Read the model definition and answer for the solid it produces. Units are mm, in the model's axes. Face numbers are marked on the shaded views. A direction names the side the tool comes from. Round coordinates to 2 decimals unless told otherwise and drop trailing zeros. Order: outer loops, then holes, each group sorted by start corner. A loop starts at its lowest first (then second) coordinate and runs counter-clockwise, first axis right, second up. Notation, with made-up numbers: (81, -26) -> (101, -26) arc R11 cw to (101, -13) -> close; hole circle Ø5 at (22.5, -23.5). An arc over 180 degrees is marked (long way). Use a Markdown table: item, result. Add a question column.
1. Consider L1, parallel to Y at x = 0, z = 8.75; L2, parallel to Z at x = -9.5, y = 2; L3, parallel to Z at x = 0.75, y = 2.25. Determine where each line is inside the solid, lowest interval first. Write a range as [from, to].
2. Section B-B, the plane z = -22.5 is taken. Give the vertices of the cut face in (x, y), then the cut area to 3 significant figures.
3. The mould has two halves that part along X. Classify the marked faces 3, 4 and 5: +X half, -X half, draft (parallel to the pull), parting line (faces both ways), or undercut.
4. For the marked faces 1 and 2, determine the directions among +Z, -Z, +X, -X, +Y, -Y from which every point of the face is accessible in a straight line to the end or side of a thin tool.
5. Given pin 1 (6 mm diameter, centred on y = 2.5, z = -12.5, fed in from +X); pin 2 (6 mm diameter, centred on x = -6, z = -24, fed in from +Y); pin 3 (1 mm diameter, centred on x = -3, z = 9.5, fed in from +Y), each flat-ended and moving along its own axis, determine where each tip first touches the part or whether it passes through.
6. Section A-A, the plane z = 15 is taken. Give the vertices of the cut face in (x, y).
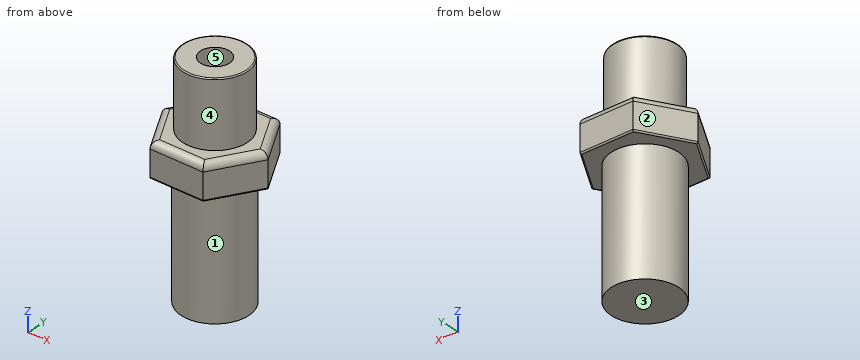
Autodesk Inventor part; units mm, degrees
ref_plane "YZ Plane" through (0, 0, 0) normal (1, 0, 0) x (0, 1, 0)
ref_plane "XZ Plane" through (0, 0, 0) normal (0, 1, 0) x (-1, 0, 0)
ref_plane "XY Plane" through (0, 0, 0) normal (0, 0, 1) x (1, 0, 0)
sketch "Sketch1" plane through (0, 0, 0) normal (0, 0, 1) x (1, 0, 0)
  line L0 (6.4577, 10.7072) -> (12.5016, -0.2389)
  line L1 (12.5016, -0.2389) -> (6.0439, -10.9461)
  line L2 (6.0439, -10.9461) -> (-6.4577, -10.7072)
  line L3 (-6.4577, -10.7072) -> (-12.5016, 0.2389)
  line L4 (-12.5016, 0.2389) -> (-6.0439, 10.9461)
  line L5 (-6.0439, 10.9461) -> (6.4577, 10.7072)
  point P0 (0, 0)
  point P1 (0, 0)
  dimension "d0" = 25.0031
extrude "Extrusion1" add sketch "Sketch1" along normal mid plane 7.874
sketch "Sketch2" plane through (0, 0, 3.937) normal (0, 0, 1) x (1, 0, 0)
  circle A0 centre (0, 0) radius 7.4676
  dimension "d3" = 14.9352
extrude "Extrusion2" add sketch "Sketch2" along normal blind 15.24
fillet "Fillet1" radius 0.254 1 edges at (-7.4676, 0, 19.177)
sketch "Sketch3" plane through (0, 0, 19.177) normal (0, 0, 1) x (1, 0, 0)
  point P0 (0, 0)
  point P1 (0, 0)
hole "Hole1" at (0, 0, 19.177) at (0, 0, 19.177) direction (0, 0, -1) diameter 6.7469 depth 15.24
sketch "Sketch4" plane through (0, 0, -3.937) normal (0, 0, -1) x (-1, 0, 0)
  circle A0 centre (0, 0) radius 7.8105
  dimension "d15" = 15.621
extrude "Extrusion3" add sketch "Sketch4" along normal blind 28.575
thread "Thread1"
thread "Thread2"
fillet "Fillet2" radius 1.5875 6 edges at (9.4796, 5.2342, 3.937) (0.2069, 10.8267, 3.937) (9.2727, -5.5925, 3.937) (-0.2069, -10.8267, 3.937) (-9.4796, -5.2342, 3.937) (-9.2727, 5.5925, 3.937)
fillet "Fillet3" radius 0.3175 6 edges at (-0.2069, -10.8267, -3.937) (9.2727, -5.5925, -3.937) (9.4796, 5.2342, -3.937) (0.2069, 10.8267, -3.937) (-9.2727, 5.5925, -3.937) (-9.4796, -5.2342, -3.937)
properties part number "Double Sided Bolt" material "Stainless Steel"
Verdict:
| question | item | result |
|---|---|---|
| 1 | L1 | y = [-7.47, -3.37], [3.37, 7.47] |
| 1 | L2 | z = [-3.94, 3.94] |
| 1 | L3 | z = [-32.51, 3.94] |
| 2 | outline | circle Ø15.62 at (0, 0) |
| 2 | area | 192 mm2 |
| 3 | face 3 | draft |
| 3 | face 4 | parting line |
| 3 | face 5 | undercut |
| 4 | face 1 | -Z |
| 4 | face 2 | +Z, -Z, -X, +Y |
| 5 | pin 1 | stops at x = 7.81 |
| 5 | pin 2 | stops at y = 7.21 |
| 5 | pin 3 | stops at y = 7.04 |
| 6 | outline | circle Ø14.94 at (0, 0); hole circle Ø6.75 at (0, 0) |
